CAD build for the part. Positions are in the model's coordinates, mm. Coordinates: 2 decimals unless noted, no trailing zeros. Loops run counter-clockwise (first coordinate to the right, second up) from the corner with the lowest first, then second, coordinate; pieces in that order, holes last. Notation, with made-up numbers: (-37, -7) -> (0, -7) arc R25 ccw to (0, 17) -> close; hole circle Ø9 at (38.25, 88.5). An arc over 180 degrees is marked (long way). Return JSON: item names as keys, results as strings. Group by question number.
(1) Saw through at C-C on y = 16. Write the cut outline in (x, z) (3 decimals).
(2) Flat gauge pins, fed straight in: pin 1 Ø7.5 at (x, z) = (19.05, 19.05) entering from -Y; pin 2 Ø5.5 at (x, z) = (-19.05, 19.05) entering from +Y; pin 3 Ø3 at (x, y) = (-11.5, -23) entering from +Z (3 decimals). Where does each tip first touch, or does it go through?
(3) Probe L1, parallel to X at y = -16, z = 19; L2, parallel to Z at x = -19, y = -4 (3 decimals); L3, parallel to Z at x = -22.5, y = 26 (3 decimals). List the from-to ranges inside material, lowest first.
(4) Saw through at B-B on z = 19.05. Write the cut outline in (x, y) (3 decimals), then the cut area to 3 significant figures.
(5) Saw through at A-A on x = 19.05. Write the cut outline in (y, z) (3 decimals).
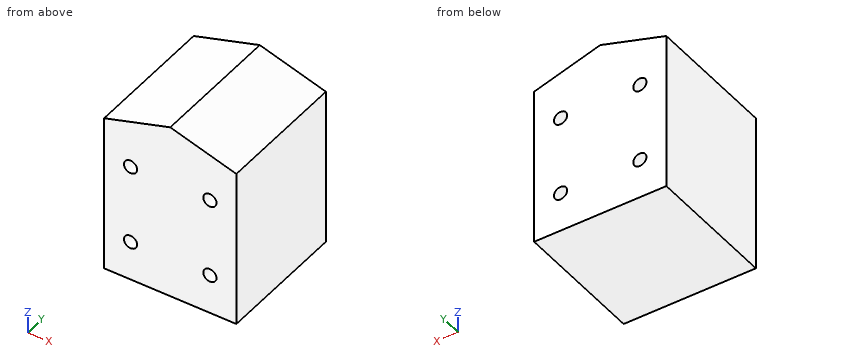
```python
from build123d import *

# Parameters (mm, degrees)
F0_W     = 63.5
F0_H     = 76.2
F1_DEPTH = 31.75
F3_DEPTH = 63.5
F5_D     = 6.35


with BuildPart() as f1:
    # F0 (on Front) → F1 (new body, symmetric)
    with BuildSketch(Plane.XZ):
        Rectangle(F0_W, F0_H)
    extrude(amount=F1_DEPTH, both=True)

    # F2 (on face) → F3 (join, through all)
    with BuildSketch(Plane.XZ.offset(31.75)):
        Polygon((0, 47.625), (-31.75, 38.1), (31.75, 38.1), align=None)
    extrude(amount=-F3_DEPTH)

    # F5 (through all)
    with Locations(Plane(origin=(0, 31.75, 0), x_dir=(-1, 0, 0), z_dir=(0, 1, 0))):
        with Locations((-19.05, 19.05), (19.05, 19.05), (-19.05, -19.05), (19.05, -19.05)):
            Hole(F5_D / 2)


solid = f1.part
```
Geometry results:
{
 "1": {"outline": "(-31.75, -38.1) -> (31.75, -38.1) -> (31.75, 38.1) -> (0, 47.625) -> (-31.75, 38.1) -> close; hole circle Ø6.35 at (-19.05, -19.05); hole circle Ø6.35 at (-19.05, 19.05); hole circle Ø6.35 at (19.05, -19.05); hole circle Ø6.35 at (19.05, 19.05)"},
 "2": {"pin 1": "y = -31.75", "pin 2": "through", "pin 3": "z = 44.625"},
 "3": {"L1": "-31.75 to -22.22, -15.88 to 15.88, 22.22 to 31.75", "L2": "-38.1 to -22.225, -15.875 to 15.875, 22.225 to 41.925", "L3": "-38.1 to 40.875"},
 "4": {"outline": "(-31.75, -31.75) -> (-22.225, -31.75) -> (-22.225, 31.75) -> (-31.75, 31.75) -> close; (-15.875, -31.75) -> (15.875, -31.75) -> (15.875, 31.75) -> (-15.875, 31.75) -> close; (22.225, -31.75) -> (31.75, -31.75) -> (31.75, 31.75) -> (22.225, 31.75) -> close", "area": "3,230 mm²"},
 "5": {"outline": "(-31.75, -38.1) -> (31.75, -38.1) -> (31.75, -22.225) -> (-31.75, -22.225) -> close; (-31.75, -15.875) -> (31.75, -15.875) -> (31.75, 15.875) -> (-31.75, 15.875) -> close; (-31.75, 22.225) -> (31.75, 22.225) -> (31.75, 41.91) -> (-31.75, 41.91) -> close"}
}
